from build123d import *

# Parameters (mm, degrees)
F1_DEPTH = 38.1
F2_W     = 25.4
F2_H     = 12.7
F3_DEPTH = 25.401


with BuildPart() as f1:
    # F0 (on Right) → F1 (new body)
    with BuildSketch(Plane.YZ):
        Polygon((25.4, 25.4), (0, 0), (25.4, 0), align=None)
    extrude(amount=-F1_DEPTH)

    # F2 (on Top) → F3 (cut, through all)
    with BuildSketch(Plane.XY):
        with Locations((-19.05, 6.35)):
            Rectangle(F2_W, F2_H)
    extrude(amount=F3_DEPTH, mode=Mode.SUBTRACT)


solid = f1.part
Here's how the part is built. I have some questions about the finished solid (model axes, mm). A direction names the side the tool comes from. Coordinates: 2 decimals unless noted, no trailing zeros. Order: outer loops, then holes, each group sorted by start corner. A loop starts at its lowest first (then second) coordinate and runs counter-clockwise, first axis right, second up.
Item 1: If we section it at D-D on y = 8.25: List the corners of the cut face in (x, z) for me, plus the area to 3 significant figures.
Result sheet:
outline: (-38.1, 0) - (-31.75, 0) - (-31.75, 8.25) - (-38.1, 8.25) - close; (-6.35, 0) - (0, 0) - (0, 8.25) - (-6.35, 8.25) - close
area: 105 mm2
Item 2: If we mould it in two halves opening along X, with no side actions, what happens to faces 3 (the face through (0, 18, 7)), 4 (the face through (-19, 12.7, 6)), 5 (the face through (-38.1, 18, 7)), 6 (the face through (-19, 15, 0))? For each: +X half, -X half, draft (parallel to the pull), parting line (faces both ways), or undercut.
Result sheet:
face 3: +X half
face 4: undercut
face 5: -X half
face 6: draft
Item 3: For P1, Ø5, axis at x = -34, y = 21.5, coming from the +Z side; P2, Ø4, axis at x = -25, z = 5.5, coming from the -Y side; P3, Ø10, axis at x = -4, z = 11, coming from the -Y side; P4, Ø12, axis at y = 8.5, z = 21.5, coming from the -X side, each with a flat end and sliding along its axis, tell me the tip position at first contact or that it passes through.
Result sheet:
P1: stops at z = 24
P2: stops at y = 12.7
P3: stops at y = 6
P4: passes through
Item 4: I need wall thicknesses on line 1 (X direction, y = 7, z = 3.25); line 2 (Y direction, x = -14.5, z = 2.5); line 3 (Z direction, x = -17, y = 17). Which ranges of each line are inside material? Lowest first, please.
Result sheet:
line 1: x = -38.1 to -31.75, -6.35 to 0
line 2: y = 12.7 to 25.4
line 3: z = 0 to 17
Item 5: For faces 1 (the face through (-6.35, 9, 3)), 2 (the face through (-19, 16, 16)), which set-ups out of +Z, -Z, +X, -X, +Y, -Y let a thin tool reach every point of the face, with its end or its side?
Result sheet:
face 1: +Z, -Z, -Y
face 2: +Z, +X, -X, -Y
Item 6: If we section it at C-C on y = 20: List the corners of the cut face in (x, z) for me, plus the area to 3 significant figures.
Result sheet:
outline: (-38.1, 0) - (0, 0) - (0, 20) - (-38.1, 20) - close
area: 762 mm2
Item 7: If we section it at B-B on z = 11.25: List the corners of the cut face in (x, y) for me, plus the area to 3 significant figures.
Result sheet:
outline: (-38.1, 11.25) - (-31.75, 11.25) - (-31.75, 12.7) - (-6.35, 12.7) - (-6.35, 11.25) - (0, 11.25) - (0, 25.4) - (-38.1, 25.4) - close
area: 502 mm2
Item 8: If we section it at A-A on y = 11.5: List the corners of the cut face in (x, z) for me, plus the area to 3 significant figures.
Result sheet:
outline: (-38.1, 0) - (-31.75, 0) - (-31.75, 11.5) - (-38.1, 11.5) - close; (-6.35, 0) - (0, 0) - (0, 11.5) - (-6.35, 11.5) - close
area: 146 mm2
